Answer from the drawing. Dimensions are ordinates in mm from the lowest x, y and z of the part. A direction names the side the tool comes from. Coordinates: 2 decimals unless noted, no trailing zeros. Order: outer loops, then holes, each group sorted by start corner. A loop starts at its lowest first (then second) coordinate and runs counter-clockwise, first axis right, second up.
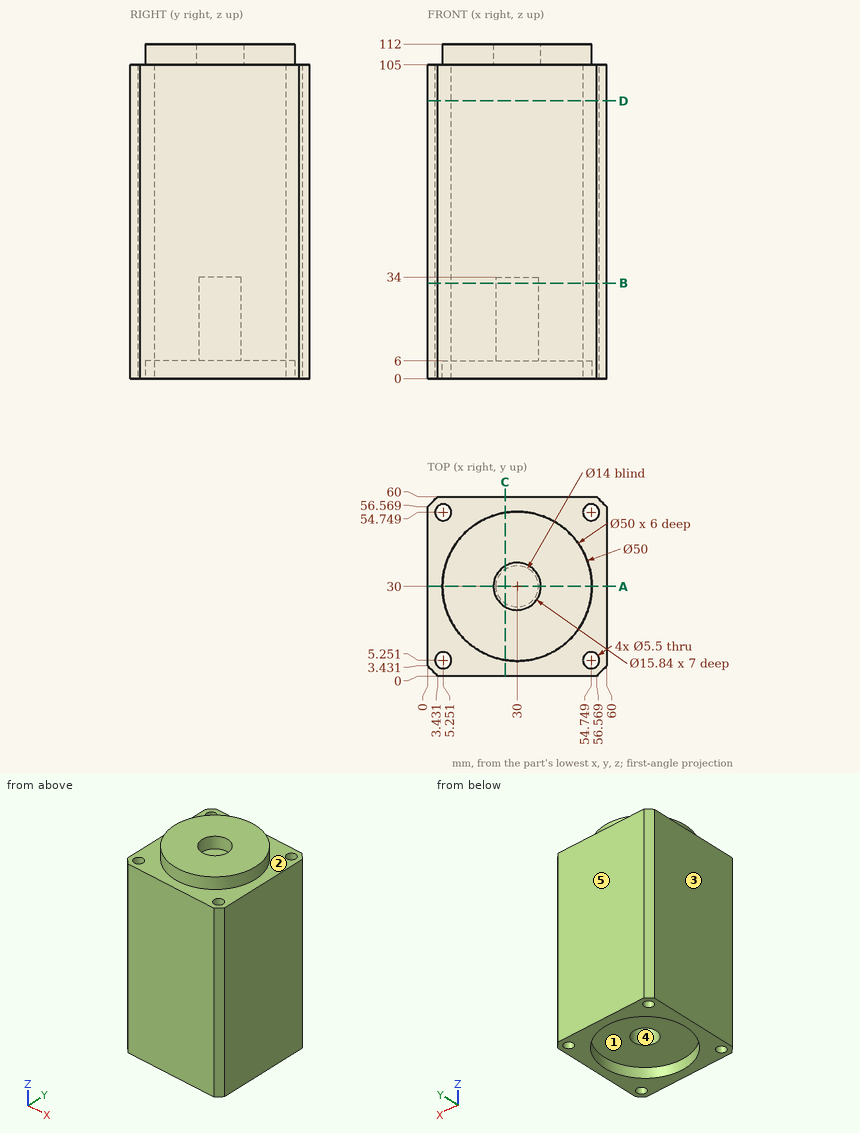
1. Consider probe 1 along X at (y, z) = (29.5, 24); probe 2 along Y at (x, z) = (30, 108.25); probe 3 along Y at (x, z) = (56.5, 22.5). Determine where each line is inside the solid, lowest interval first.
2. The part is cut by section A-A (y = 30). Determine the outline of the cut face in (x, z), plus the area to 3 significant figures.
3. The part is cut by section C-C (x = 26). Determine the outline of the cut face in (y, z) (1 decimal), plus the area to 3 significant figures.
4. The mould has two halves that part along X. Classify the marked faces 1, 2 and 3: released by +X, released by -X, zero draft, split by the parting line, or undercut.
5. The part is cut by section B-B (z = 32). Determine the outline of the cut face in (x, y), plus the area to 3 significant figures.
6. Flat-ended cylindrical pins translate along their axes: pin 1 (3.5 mm diameter, centred on x = 54.75, y = 54.75, fed in from -Z); pin 2 (2 mm diameter, centred on y = 18.5, z = 65.5, fed in from -X); pin 3 (4 mm diameter, centred on x = 30.5, y = 31.5, fed in from +Z); pin 4 (9.5 mm diameter, centred on x = 30, y = 30, fed in from -Z). Find the tip coordinate at first contact, or state that the pin passes through.
7. For the marked faces 4 and 5, determine the directions among +Z, -Z, +X, -X, +Y, -Y from which every point of the face is accessible in a straight line to the end or side of a thin tool.
8. The part is cut by section D-D (z = 93). Determine the outline of the cut face in (x, y).
Worked out:
1. probe 1: x = 0 to 23.02, 36.98 to 60
1. probe 2: y = 5 to 22.08, 37.92 to 55
1. probe 3: y = 0 to 3.13, 7.37 to 52.63, 56.87 to 60
2. outline: (0, 0) - (5, 0) - (5, 6) - (23, 6) - (23, 34) - (37, 34) - (37, 6) - (55, 6) - (55, 0) - (60, 0) - (60, 105) - (55, 105) - (55, 112) - (37.92, 112) - (37.92, 105) - (22.08, 105) - (22.08, 112) - (5, 112) - (5, 105) - (0, 105) - close
2. area: 5,850 mm2
3. outline: (0, 0) - (5.3, 0) - (5.3, 6) - (24.3, 6) - (24.3, 34) - (35.7, 34) - (35.7, 6) - (54.7, 6) - (54.7, 0) - (60, 0) - (60, 105) - (54.7, 105) - (54.7, 112) - (36.8, 112) - (36.8, 105) - (23.2, 105) - (23.2, 112) - (5.3, 112) - (5.3, 105) - (0, 105) - close
3. area: 5,930 mm2
4. face 1: undercut
4. face 2: zero draft
4. face 3: released by -X
5. outline: (0, 3.43) - (3.43, 0) - (56.57, 0) - (60, 3.43) - (60, 56.57) - (56.57, 60) - (3.43, 60) - (0, 56.57) - close; hole circle Ø5.5 at (5.25, 5.25); hole circle Ø5.5 at (5.25, 54.75); hole circle Ø14 at (30, 30); hole circle Ø5.5 at (54.75, 5.25); hole circle Ø5.5 at (54.75, 54.75)
5. area: 3,330 mm2
6. pin 1: passes through
6. pin 2: stops at x = 0
6. pin 3: stops at z = 105
6. pin 4: stops at z = 34
7. face 4: -Z
7. face 5: +Z, -Z, +X, -X, +Y
8. outline: (0, 3.43) - (3.43, 0) - (56.57, 0) - (60, 3.43) - (60, 56.57) - (56.57, 60) - (3.43, 60) - (0, 56.57) - close; hole circle Ø5.5 at (5.25, 5.25); hole circle Ø5.5 at (5.25, 54.75); hole circle Ø5.5 at (54.75, 5.25); hole circle Ø5.5 at (54.75, 54.75)
